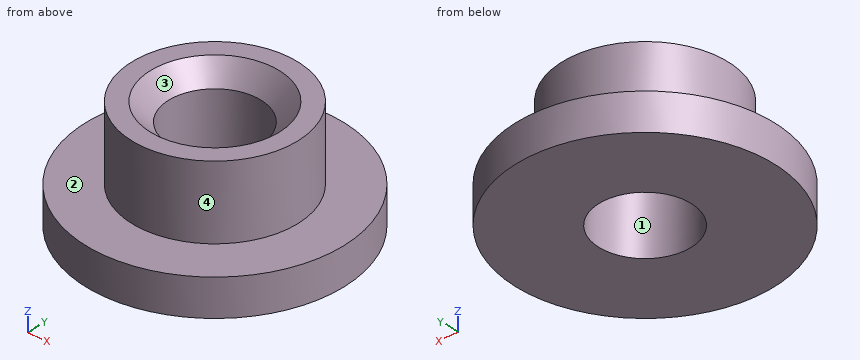
```python
from build123d import *

# Parameters (mm, degrees)
F0_R     = 2.25
F0_R_2   = 1.25
F1_DEPTH = 2
F2_SIZE  = 0.5
F3_R     = 3.5
F3_R_2   = 1.25
F4_DEPTH = 1


with BuildPart() as f1:
    # F0 (on Top) → F1 (new body)
    with BuildSketch(Plane.XY):
        Circle(F0_R)
        Circle(F0_R_2, mode=Mode.SUBTRACT)
    extrude(amount=F1_DEPTH)

    # F2
    f2_edges = [f1.edges().sort_by_distance(p)[0] for p in [
        (-1.25, 0, 2),
    ]]
    chamfer(f2_edges, length=F2_SIZE)

    # F3 (on face) → F4 (join)
    with BuildSketch(Plane(origin=(0, 0, 0), x_dir=(1, 0, 0), z_dir=(0, 0, -1))):
        Circle(F3_R)
        Circle(F3_R_2, mode=Mode.SUBTRACT)
    extrude(amount=F4_DEPTH)


solid = f1.part
```
Geometry check sheet. Reference: the model listing, model coordinates, mm. Face numbers are marked on the shaded views. Round coordinates to 2 decimals unless told otherwise and drop trailing zeros. Order: outer loops, then holes, each group sorted by start corner. A loop starts at its lowest first (then second) coordinate and runs counter-clockwise, first axis right, second up. Notation, with made-up numbers: (-22, 71.25) - (-14, 71.25) arc R20 ccw to (-14, 99.25) - close; hole circle Ø4 at (32, 11.5). An arc over 180 degrees is marked (long way). Use a Markdown table: item, result. Add a question column.
(1) Depth check by flat-ended pin: pin 1 (1 mm diameter, centred on x = -1.5, z = -0.5, fed in from -Y); pin 2 (1.5 mm diameter, centred on y = 1, z = 0, fed in from -X); pin 3 (1.5 mm diameter, centred on y = 0.5, z = 1.5, fed in from -X). Enter the tip coordinate at first touch or a pass-through.
(2) Sectioned sample at D-D, the plane y = 2.5. Enter the section's corners in (x, z), and give its area (3 significant figures).
(3) Sectioned sample at C-C, the plane z = 1.2. Enter the section's corners in (x, y).
(4) Sectioned sample at A-A, the plane y = 0. Enter the section's corners in (x, z).
(5) Material ranges on line 1 along Y through (x, z) = (0, -0.2); line 2 along Y through (x, z) = (0, 0.05), recorded low to high. Write a range as [from, to].
(6) Release check for a two-part mould opening along X. For the marked faces 1, 2, 3 and 4 record: pulls with the +X half, pulls with the -X half, needs draft (parallel to the pull), parting line crosses it, or undercut.
Answers below:
| question | item | result |
|---|---|---|
| 1 | pin 1 | y = -3.35 |
| 1 | pin 2 | x = -3.49 |
| 1 | pin 3 | x = -2.25 |
| 2 | outline | (-2.45, -1) - (2.45, -1) - (2.45, 0) - (-2.45, 0) - close |
| 2 | area | 4.90 mm² |
| 3 | outline | circle Ø4.5 at (0, 0); hole circle Ø2.5 at (0, 0) |
| 4 | outline | (-3.5, -1) - (-1.25, -1) - (-1.25, 1.5) - (-1.75, 2) - (-2.25, 2) - (-2.25, 0) - (-3.5, 0) - close; (1.25, -1) - (3.5, -1) - (3.5, 0) - (2.25, 0) - (2.25, 2) - (1.75, 2) - (1.25, 1.5) - close |
| 5 | line 1 | [-3.5, -1.25], [1.25, 3.5] |
| 5 | line 2 | [-2.25, -1.25], [1.25, 2.25] |
| 6 | face 1 | undercut |
| 6 | face 2 | needs draft |
| 6 | face 3 | undercut |
| 6 | face 4 | parting line crosses it |
